Here's how the part is built. I have some questions about the finished solid (model axes, mm). Round coordinates to 2 decimals unless told otherwise and drop trailing zeros. Loops run counter-clockwise (first coordinate to the right, second up) from the corner with the lowest first, then second, coordinate; pieces in that order, holes last. Notation, with made-up numbers: M 49.25,49 L 85.25,49 A30 ccw 85.25,74 Z; hole C 47.25,-35.5 d11. An arc over 180 degrees is marked long. One line per question, with ' | ' between items. Start each with the question number.
```python
from build123d import *

# Parameters (mm, degrees)
BOSS_EXTRUDE1_DEPTH = 1
FILLET1_R           = 1


with BuildPart() as part:
    # Sketch1 → Boss-Extrude1 (new body)
    with BuildSketch(Plane(origin=(0, 0, 0), x_dir=(1, 0, 0), z_dir=(0, 1, 0))):
        Polygon((0, 0), (0, 27.5), (69.5, 27.5), (69.5, -27), (-22.5, -27), (-22.5, -7), (-15, -7), (-15, 0), align=None)
    extrude(amount=BOSS_EXTRUDE1_DEPTH)

    # Fillet1
    fillet1_edges = [part.edges().sort_by_distance(p)[0] for p in [
        (0, 0.5, 0),
        (-15, 0.5, 7),
    ]]
    fillet(fillet1_edges, radius=FILLET1_R)


solid = part.part
```
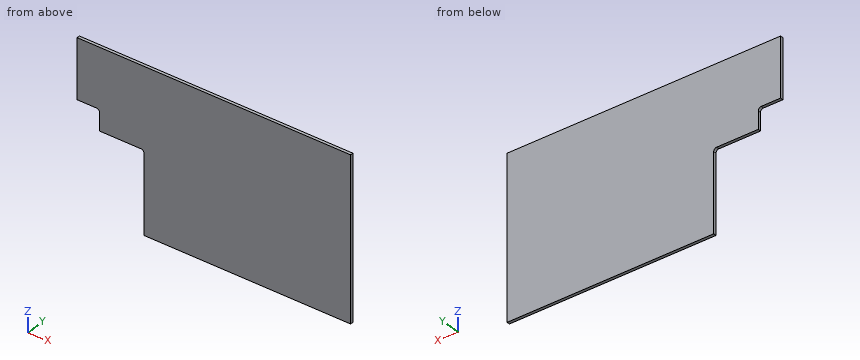
1) I'm going to push flat-ended pins straight in: pin 1 Ø0.5 at (y, z) = (0.5, -21) entering from -X; pin 2 Ø0.5 at (y, z) = (0.5, 2.5) entering from -X. Where does each tip first touch, or does it pass through?
2) Imagine slicing it at B-B (x = -8). Write out the boundary of the cut face in (y, z).
3) Imagine slicing it at A-A (y = 0.6). Write out the boundary of the cut face in (x, z).
4) Imagine slicing it at C-C (z = -12). Write out the boundary of the cut face in (x, y).
5) Please list where these lines run through material, in increasing order: L1, parallel to X at y = 0.7, z = -14; L2, parallel to X at y = 0.55, z = 4.5; L3, parallel to Z at x = -17, y = 0.85. Write a range as from..to.
Results are:
1) pin 1: x = 0 | pin 2: x = -15
2) outline: M 0,0 L 1,0 L 1,27 L 0,27 Z
3) outline: M -22.5,7 L -16,7 A1 cw -15,6 L -15,0 L -1,0 A1 cw 0,-1 L 0,-27.5 L 69.5,-27.5 L 69.5,27 L -22.5,27 Z
4) outline: M 0,0 L 69.5,0 L 69.5,1 L 0,1 Z
5) L1: 0..69.5 | L2: -15..69.5 | L3: 7..27
